Can you work these out from the drawing? Everything is in mm from the part's minimum corner. A direction names the side the tool comes from. Coordinates: 2 decimals unless noted, no trailing zeros. Loops run counter-clockwise (first coordinate to the right, second up) from the corner with the lowest first, then second, coordinate; pieces in that order, holes last.
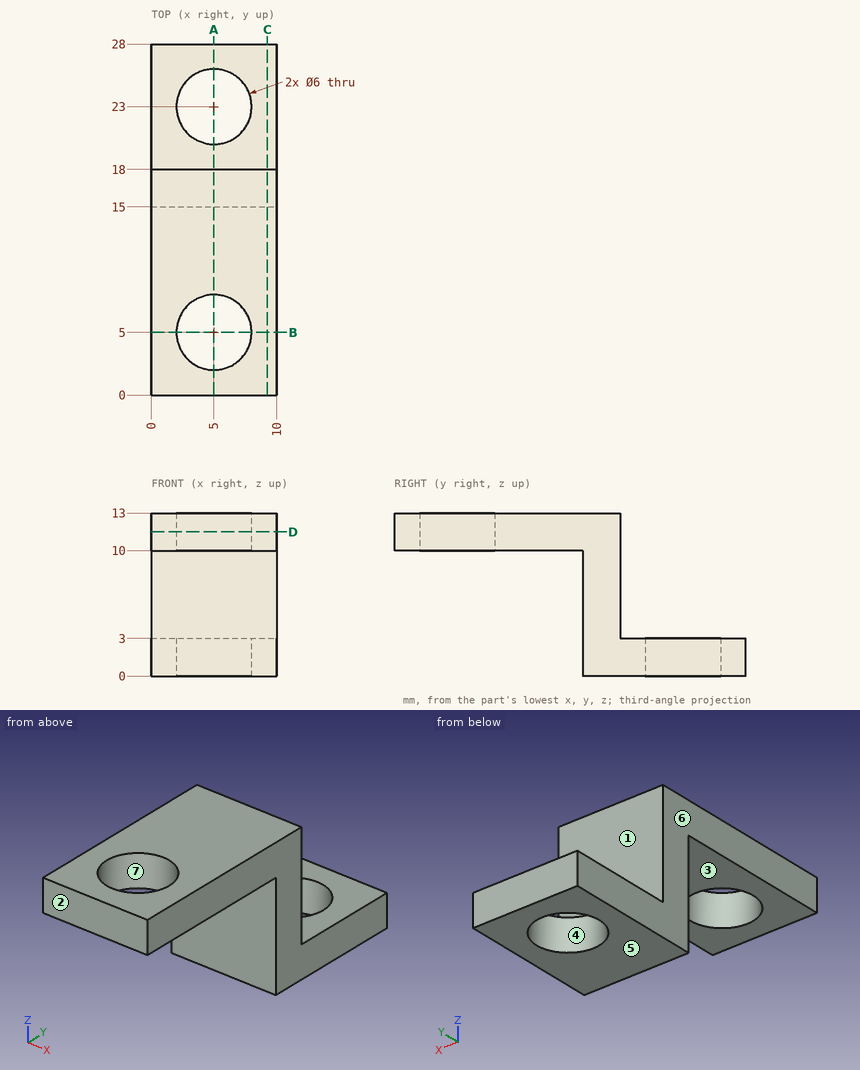
Item 1: On a 3-axis mill with a long thin cutter (end or side, diameter ignored), from which of +Z, -Z, +X, -X, +Y, -Y can I reach the whole of each face in a straight line? I mean the marked faces 1, 2 and 3. Say none if no direction works.
Results are:
face 1: +Z, +X, -X, +Y
face 2: +Z, -Z, +X, -X, -Y
face 3: -Z, +X, -X, -Y
Item 2: Suppose I cut it at A-A, the plane x = 5. Please give me the cut outline in (y, z).
Results are:
outline: (0, 10) - (2, 10) - (2, 13) - (0, 13) - close; (8, 10) - (15, 10) - (15, 0) - (20, 0) - (20, 3) - (18, 3) - (18, 13) - (8, 13) - close; (26, 0) - (28, 0) - (28, 3) - (26, 3) - close
Item 3: I'm going to push flat-ended pins straight in: P1, Ø1, axis at x = 7, z = 10.5, coming from the +Y side; P2, Ø5, axis at x = 5, y = 23, coming from the -Z side; P3, Ø5, axis at x = 4.5, y = 22, coming from the +Z side; P4, Ø5, axis at x = 5, y = 4, coming from the -Z side. Where does each tip first touch, or does it pass through?
Results are:
P1: stops at y = 18
P2: passes through
P3: stops at z = 3
P4: stops at z = 10
Item 4: I need wall thicknesses on line 1 along Y through (x, z) = (5, 11.5); line 2 along Y through (x, z) = (5, 2); line 3 along Z through (x, y) = (1.25, 22.5). Which ranges of each line are inside material? Lowest first, please.
Results are:
line 1: y = 0 to 2, 8 to 18
line 2: y = 15 to 20, 26 to 28
line 3: z = 0 to 3
Item 5: Suppose I cut it at B-B, the plane y = 5. Please give me the cut outline in (x, z), plus the area to 3 significant figures.
Results are:
outline: (0, 10) - (2, 10) - (2, 13) - (0, 13) - close; (8, 10) - (10, 10) - (10, 13) - (8, 13) - close
area: 12.0 mm2
Item 6: We'd pull the mould along X, two halves only. Please class the marked faces 4, 5, 6 and 7: +X half, -X half, draft (parallel to the pull), parting line (faces both ways), or undercut.
Results are:
face 4: undercut
face 5: draft
face 6: -X half
face 7: undercut
Item 7: Suppose I cut it at D-D, the plane z = 11.5. Please give me the cut outline in (x, y).
Results are:
outline: (0, 0) - (10, 0) - (10, 18) - (0, 18) - close; hole circle Ø6 at (5, 5)
Item 8: Suppose I cut it at C-C, the plane x = 9.25. Please give me the cut outline in (y, z).
Results are:
outline: (0, 10) - (15, 10) - (15, 0) - (28, 0) - (28, 3) - (18, 3) - (18, 13) - (0, 13) - close
